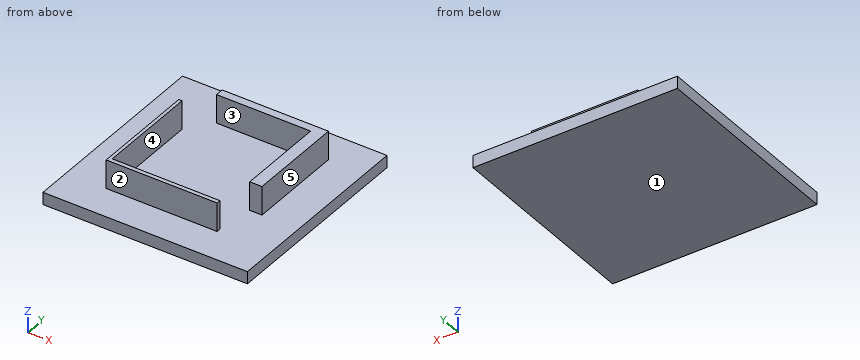
```python
from build123d import *

# Parameters (mm, degrees)
F1_DEPTH = 5
F0_W     = 25
F0_H     = 25
F2_DEPTH = 1.5
F3_DEPTH = 5


with BuildPart() as f1:
    # F0 (on Top) → F1 (new body)
    with BuildSketch(Plane.XY):
        Polygon((-4.457476, 8.541189), (-17.457476, 8.541189), (-17.457476, 7.541189), (-5.957476, 7.541189), (-5.957476, -3.366469), (-4.457476, -3.366469), align=None)
    extrude(amount=F1_DEPTH)

    # F0 (on Top) → F2 (join)
    with BuildSketch(Plane.XY):
        with Locations((-12.5, 0)):
            Rectangle(F0_W, F0_H)
        Polygon((-20.116894, 4.669981), (-19.716894, 4.669981), (-19.716894, -7.830019), (-6.561746, -7.830019), (-6.561746, -8.330019), (-20.116894, -8.330019), align=None, mode=Mode.SUBTRACT)
        Polygon((-17.457476, 7.541189), (-17.457476, 8.541189), (-4.457476, 8.541189), (-4.457476, -3.366469), (-5.957476, -3.366469), (-5.957476, 7.541189), align=None, mode=Mode.SUBTRACT)
    extrude(amount=F2_DEPTH)

    # F0 (on Top) → F3 (join)
    with BuildSketch(Plane.XY):
        Polygon((-19.716894, -7.830019), (-19.716894, 4.669981), (-20.116894, 4.669981), (-20.116894, -8.330019), (-6.561746, -8.330019), (-6.561746, -7.830019), align=None)
    extrude(amount=F3_DEPTH)


solid = f1.part
```
For this review, take the finished solid that the model builds, in its own axes (mm). Face numbers are marked on the shaded views. A direction names the side the tool comes from. Coordinates: 2 decimals unless noted, no trailing zeros. Write each loop counter-clockwise with the first axis right and the second up, starting at its lowest first coordinate (ties: lowest second). Pieces come first, ordered by that corner, then holes. Notation, with made-up numbers: (31.5, 40.5) - (61.5, 40.5) arc R19 ccw to (61.5, 66.5) - close; hole circle Ø1 at (9, 63). An arc over 180 degrees is marked (long way). Answer in a Markdown table with one row per item. Add a question column.
Q1. Draft analysis for pull direction Y (two halves, no side actions). For the marked faces 1, 2 and 3, state which applies: +Y half, -Y half, draft (parallel to the pull), parting line (faces both ways), or undercut.
Q2. For P1, Ø3, axis at y = 4, z = 4, coming from the +X side; P2, Ø1, axis at y = -4.5, z = 4, coming from the +X side; P3, Ø2, axis at y = 7, z = 3, coming from the -X side, all flat-tipped, find the tip position at first contact; note any pin that passes through.
Q3. We need section B-B, the plane x = -7.25. State the section outline as (y, z) points, and give its area (4 significant figures).
Q4. We need section D-D, the plane y = 2. State the section outline as (x, z) points, and give its area (4 significant figures).
Q5. We need section A-A, the plane z = 2.85. State the section outline as (x, y) points.
Q6. For probe 1 along Y at (x, z) = (-11.5, 2.6); probe 2 along X at (y, z) = (1.5, 2.35); probe 3 along Y at (x, z) = (-19, 2.4), list the stretches that pass through material, from the lowest coordinate up.
Q7. We need section C-C, the plane y = -5. State the section outline as (x, z) points.
Q8. Tool access review of the marked faces 4 and 5: name each direction out of +Z, -Z, +X, -X, +Y, -Y from which nothing blocks a thin tool from reaching the whole face with its end or side.
Answer list:
| question | item | result |
|---|---|---|
| 1 | face 1 | draft |
| 1 | face 2 | -Y half |
| 1 | face 3 | undercut |
| 2 | P1 | stops at x = -4.46 |
| 2 | P2 | stops at x = -19.72 |
| 2 | P3 | stops at x = -17.46 |
| 3 | outline | (-12.5, 0) - (12.5, 0) - (12.5, 1.5) - (8.54, 1.5) - (8.54, 5) - (7.54, 5) - (7.54, 1.5) - (-7.83, 1.5) - (-7.83, 5) - (-8.33, 5) - (-8.33, 1.5) - (-12.5, 1.5) - close |
| 3 | area | 42.75 mm2 |
| 4 | outline | (-25, 0) - (0, 0) - (0, 1.5) - (-4.46, 1.5) - (-4.46, 5) - (-5.96, 5) - (-5.96, 1.5) - (-19.72, 1.5) - (-19.72, 5) - (-20.12, 5) - (-20.12, 1.5) - (-25, 1.5) - close |
| 4 | area | 44.15 mm2 |
| 5 | outline | (-20.12, -8.33) - (-6.56, -8.33) - (-6.56, -7.83) - (-19.72, -7.83) - (-19.72, 4.67) - (-20.12, 4.67) - close; (-17.46, 7.54) - (-5.96, 7.54) - (-5.96, -3.37) - (-4.46, -3.37) - (-4.46, 8.54) - (-17.46, 8.54) - close |
| 6 | probe 1 | y = -8.33 to -7.83, 7.54 to 8.54 |
| 6 | probe 2 | x = -20.12 to -19.72, -5.96 to -4.46 |
| 6 | probe 3 | y = -8.33 to -7.83 |
| 7 | outline | (-25, 0) - (0, 0) - (0, 1.5) - (-19.72, 1.5) - (-19.72, 5) - (-20.12, 5) - (-20.12, 1.5) - (-25, 1.5) - close |
| 8 | face 4 | +Z, +Y |
| 8 | face 5 | +Z, +X, +Y, -Y |
